Part model, mm, in its own coordinate system. A direction names the side the tool comes from. Give positions to 0.01 mm unless a question says otherwise; leave off trailing zeros. Order: outer loops, then holes, each group sorted by start corner. A loop starts at its lowest first (then second) coordinate and runs counter-clockwise, first axis right, second up. Notation, with made-up numbers: (-38, 34) -> (4, 34) arc R28 cw to (4, 69) -> close; hole circle Ø6 at (47, 88.5). An arc over 180 degrees is marked (long way). Write item = value, one per line. Start each with the question number.
(1) Which spindle directions (+Z, -Z, +X, -X, +Y, -Y) get a long thin tool onto all of the face, cutting with end or side? Do faces 1 (the flat face through (-29.1, -25.7, 3)), 2 (the cylindrical face through (26, -29, 4)). Say none if no direction does.
(2) Saw through at D-D, the plane y = -29. State how many separate pieces and enclosed holes the cut face has, then the cut area to 3 significant figures.
(3) Saw through at C-C, the plane z = 31. List the corners of the cut face in (x, y).
(4) Probe line 1 along X through (y, z) = (29, 4); line 2 along Y through (x, z) = (29, 1.8); line 3 along X through (y, z) = (29, 1). List the from-to ranges inside material, lowest first. Write a range as from..to.
(5) Two-plate mould, pull along X, no slides. Class faces 3 (the cylindrical face through (25, -26, 1)), 4 (the flat face through (28.9, 32.3, 3)), 5 (the flat face through (25, 1, 5.5)), 6 (the conical face through (-16.9, -12.96, 45.56)): pulls with the +X half, pulls with the -X half, needs draft (parallel to the pull), parting line crosses it, or undercut.
(6) Flat gauge pins, fed straight in: pin 1 (5 mm diameter, centred on x = 29.5, y = 31, fed in from -Z); pin 2 (13 mm diameter, centred on x = -29, y = 29, fed in from +Z); pin 3 (10 mm diameter, centred on x = -4.5, y = -2.5, fed in from -Z). Where does each tip first touch, or does it go through?
from build123d import *

# Parameters (mm, degrees)
F0_R           = 22.25
F0_R_2         = 21.25
F1_DEPTH       = 85.5
F1_TAPER       = 1.2
F2_T           = -4
F0_R_3         = 58.5
F0_R_4         = 3
F3_DEPTH       = 5.5
F4_R           = 5.49999
F5_D           = 6
F5_DEPTH       = 5
F5_CBORE_D     = 10
F5_CBORE_DEPTH = 3
F5_TIP         = 1.8025818571
F6_R           = 1
F7_R           = 3


# Not quite as in the source:
# - a fillet or chamfer is up to 0.001 mm smaller than in the source, because OpenCascade refuses the exact size


with BuildPart() as f1:
    # F0 (on Top) → F1 (new body)
    with BuildSketch(Plane.XY):
        Circle(F0_R)
        Circle(F0_R_2, mode=Mode.SUBTRACT)
        Circle(F0_R_2)
    extrude(amount=F1_DEPTH, taper=F1_TAPER)

    # F2
    f2_openings = [f1.faces().sort_by_distance(p)[0] for p in [
        (0, 0, 0),
    ]]
    offset(amount=F2_T, openings=f2_openings)

    # F0 (on Top) → F3 (join)
    with BuildSketch(Plane.XY):
        Circle(F0_R_3)
        with Locations((-29, -29)):
            Circle(F0_R_4, mode=Mode.SUBTRACT)
        with Locations((29, -29)):
            Circle(F0_R_4, mode=Mode.SUBTRACT)
        with Locations((-29, 29)):
            Circle(F0_R_4, mode=Mode.SUBTRACT)
        Circle(F0_R, mode=Mode.SUBTRACT)
        with Locations((29, 29)):
            Circle(F0_R_4, mode=Mode.SUBTRACT)
        Circle(F0_R)
        Circle(F0_R_2, mode=Mode.SUBTRACT)
    extrude(amount=F3_DEPTH)

    # F4 (radius 5.5 in the source; OpenCascade refuses exactly that, so slightly less here)
    f4_edges = [f1.edges().sort_by_distance(p)[0] for p in [
        (-58.5, 0, 0),
    ]]
    fillet(f4_edges, radius=F4_R)

    # F5
    with Locations(Plane(origin=(0, 0, 0), x_dir=(1, 0, 0), z_dir=(0, 0, -1))):
        with Locations((29, -29), (-29, -29), (-29, 29), (29, 29)):
            CounterBoreHole(F5_D / 2, F5_CBORE_D / 2, F5_CBORE_DEPTH, depth=F5_DEPTH)
            with Locations((0, 0, -(F5_DEPTH + F5_TIP / 2))):  # 118° drill point
                Cone(0, F5_D / 2, F5_TIP, mode=Mode.SUBTRACT)

    # F6
    f6_edges = [f1.edges().sort_by_distance(p)[0] for p in [
        (-20.45903, 0, 85.5),
    ]]
    fillet(f6_edges, radius=F6_R)

    # F7
    f7_edges = [f1.edges().sort_by_distance(p)[0] for p in [
        (-18.249123, 0, 0),
    ]]
    fillet(f7_edges, radius=F7_R)


solid = f1.part
Results list:
q1.face_1 = -Z
q1.face_2 = +Z, -Z
q2.separate_pieces = 3
q2.enclosed_holes = 0
q2.area = 454 mm^2
q3.outline = circle Ø43.2 at (0, 0); hole circle Ø35.2 at (0, 0)
q4.line_1 = -50.57..-32, -26..26, 32..50.57
q4.line_2 = -49.15..-34, -24..24, 34..49.15
q4.line_3 = -48.1..-34, -24..24, 34..48.1
q5.face_3 = undercut
q5.face_4 = undercut
q5.face_5 = needs draft
q5.face_6 = parting line crosses it
q6.pin_1 = 3
q6.pin_2 = 5.5
q6.pin_3 = 81.5
